from build123d import *

# Parameters (mm, degrees)
SKETCH_1_W          = 200
SKETCH_1_H          = 125
EXTRUDE_1_DEPTH     = 3
SKETCH_2_R          = 4
SKETCH_2_R_2        = 2
EXTRUDE_2_DEPTH     = 28
SKETCH_3_R          = 1.25
CUT_EXTRUDE_1_DEPTH = 10
SKETCH_4_R          = 2
CUT_EXTRUDE_2_DEPTH = 122.203341538
SKETCH_5_R          = 3
EXTRUDE_3_DEPTH     = 8
SKETCH_6_R          = 1.5
CUT_EXTRUDE_3_DEPTH = 8
FILLET_1_R          = 10
RIB_1_REACH         = 205.812
SKETCH_9_WALL_W     = 423.76696313
SKETCH_9_WALL_H     = 5
RIB_2_REACH         = 205.812
SKETCH_10_WALL_W    = 423.76696313
SKETCH_10_WALL_H    = 5
SKETCH_13_R         = 4
EXTRUDE_4_DEPTH     = 8
FILLET_3_R          = 10
SKETCH_14_R         = 1.25
CUT_EXTRUDE_4_DEPTH = 8


with BuildPart() as part:
    # 草图1 → 凸台-拉伸1 (new body)
    with BuildSketch(Plane.XY):
        Rectangle(SKETCH_1_W, SKETCH_1_H)
    extrude(amount=EXTRUDE_1_DEPTH)

    # 草图2 → 凸台-拉伸2 (add)
    with BuildSketch(Plane.XY.offset(3)):
        with Locations(Location((-91.5, 19, 0), (0, 0, 180))):
            Circle(SKETCH_2_R)
        with Locations(Location((-68.5, 19, 0), (0, 0, 180))):
            Circle(SKETCH_2_R_2)
        with Locations(Location((-80, 0, 0), (0, 0, 180))):
            Circle(SKETCH_2_R)
    extrude(amount=EXTRUDE_2_DEPTH)

    # 草图3 → 切除-拉伸1 (cut)
    with BuildSketch(Plane.XY.offset(31)):
        with Locations((-91.5, 19)):
            Circle(SKETCH_3_R)
        with Locations((-68.5, 19)):
            Circle(SKETCH_3_R)
    extrude(amount=-CUT_EXTRUDE_1_DEPTH, mode=Mode.SUBTRACT)

    # 草图4 → 切除-拉伸2 (cut, through all)
    with BuildSketch(Plane.XY.offset(3)):
        with Locations((15.5, 41)):
            Circle(SKETCH_4_R)
        with Locations((15.5, -41)):
            Circle(SKETCH_4_R)
        with Locations((5.5, 41)):
            Circle(SKETCH_4_R)
        with Locations((-4.5, 41)):
            Circle(SKETCH_4_R)
        with Locations((-14.5, -41)):
            Circle(SKETCH_4_R)
        with Locations((-24.5, -41)):
            Circle(SKETCH_4_R)
        with Locations((-4.5, -41)):
            Circle(SKETCH_4_R)
    extrude(amount=-CUT_EXTRUDE_2_DEPTH, mode=Mode.SUBTRACT)

    # 草图5 → 凸台-拉伸3 (add)
    with BuildSketch(Plane.XY.offset(3)):
        with Locations(Location((28.77, 42.73, 0), (0, 0, 180))):
            Circle(SKETCH_5_R)
        with Locations(Location((28.77, -42.73, 0), (0, 0, 180))):
            Circle(SKETCH_5_R)
        with Locations(Location((91.23, -42.73, 0), (0, 0, 180))):
            Circle(SKETCH_5_R)
        with Locations(Location((91.23, 42.73, 0), (0, 0, 180))):
            Circle(SKETCH_5_R)
    extrude(amount=EXTRUDE_3_DEPTH)

    # 草图6 → 切除-拉伸3 (cut)
    with BuildSketch(Plane.XY.offset(11)):
        with Locations((28.77, 42.73)):
            Circle(SKETCH_6_R)
        with Locations((91.23, 42.73)):
            Circle(SKETCH_6_R)
        with Locations((28.77, -42.73)):
            Circle(SKETCH_6_R)
        with Locations((91.23, -42.73)):
            Circle(SKETCH_6_R)
    extrude(amount=-CUT_EXTRUDE_3_DEPTH, mode=Mode.SUBTRACT)

    # 圆角1
    fillet_1_edges = [part.edges().sort_by_distance(p)[0] for p in [
        (100, -62.5, 1.5),
        (-100, -62.5, 1.5),
        (-100, 62.5, 1.5),
        (100, 62.5, 1.5),
    ]]
    fillet(fillet_1_edges, radius=FILLET_1_R)

    # 草图9 wall → 筋1 (add, up to next)
    with BuildSketch(Plane(origin=(-91.5, 28, 8), x_dir=(0, -0.707106781187, 0.707106781187), z_dir=(0, 0.707106781187, 0.707106781187)), mode=Mode.PRIVATE) as rib_1_sk1:
        Rectangle(SKETCH_9_WALL_W, SKETCH_9_WALL_H)
    rib_1_tool1 = extrude(rib_1_sk1.sketch, amount=-RIB_1_REACH, mode=Mode.PRIVATE) - part.part
    add(rib_1_tool1.solids().sort_by_distance((-91.5, 28, 8))[0])

    # 草图10 wall → 筋2 (add, up to next)
    with BuildSketch(Plane(origin=(-91.5, 10, 8), x_dir=(0, -0.707106781187, -0.707106781187), z_dir=(0, -0.707106781187, 0.707106781187)), mode=Mode.PRIVATE) as rib_2_sk1:
        Rectangle(SKETCH_10_WALL_W, SKETCH_10_WALL_H)
    rib_2_tool1 = extrude(rib_2_sk1.sketch, amount=-RIB_2_REACH, mode=Mode.PRIVATE) - part.part
    add(rib_2_tool1.solids().sort_by_distance((-91.5, 10, 8))[0])

    # 草图13 → 凸台-拉伸4 (add)
    with BuildSketch(Plane.XY.offset(3)):
        with Locations(Location((-68.5, 19, 0), (0, 0, 180))):
            Circle(SKETCH_13_R)
    extrude(amount=EXTRUDE_4_DEPTH)

    # 圆角3
    # the kernel refuses this fillet: 10 mm, written as the material it adds along each edge
    with BuildSketch(Plane(origin=(-68.5, 19, 11), x_dir=(-1, 0, 0), z_dir=(0, -1, 0))) as fillet_3_piece_1:
        with BuildLine():
            CenterArc((12, -6), FILLET_3_R, 143.130102354, 36.869897646)
            Line((2, -6), (1.8, -6))
            Line((1.8, -6), (1.8, 0))
            Line((1.8, 0), (2, 0.2))
            ThreePointArc((2, 0.2), (3, 0.2), (3.84, 0.12))
            Line((3.84, 0.12), (4, 0))
        make_face()
    revolve(axis=Axis((-68.5, 19, 11), (0, 0, -1)))

    # 草图14 → 切除-拉伸4 (cut)
    with BuildSketch(Plane.XY.offset(31)):
        with Locations((-80, 0)):
            Circle(SKETCH_14_R)
    extrude(amount=-CUT_EXTRUDE_4_DEPTH, mode=Mode.SUBTRACT)


solid = part.part
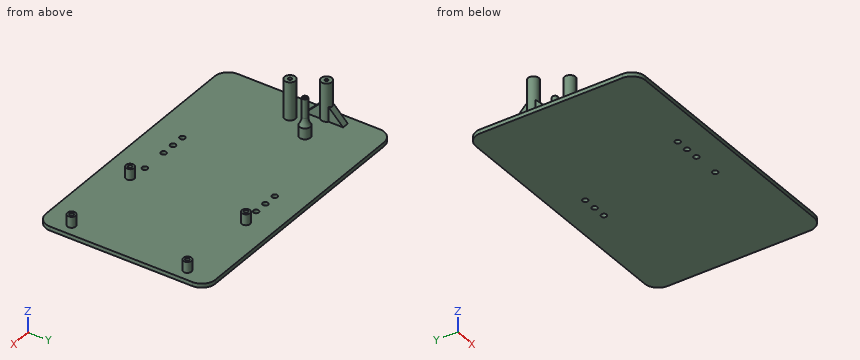
Build history of the part. All positions in model axes, mm. Round coordinates to 2 decimals unless told otherwise and drop trailing zeros. Write each loop counter-clockwise with the first axis right and the second up, starting at its lowest first coordinate (ties: lowest second). Pieces come first, ordered by that corner, then holes. Notation, with made-up numbers: M 64,30 L 112,30 A21 ccw 112,51 Z; hole C -23.5,-33 d8. An arc over 180 degrees is marked long. Answer as a JSON object with one key per item and string values. Group by question number.
(1) Cut at C-C (y = -27). Give the cut face in (x, z).
(2) Cut at A-A (z = 29). Give the cut face in (x, y).
(3) Cut at D-D (x = -35). Give the cut face in (y, z), and give its area (3 significant figures).
(4) Flat gauge pins, fed straight in: pin 1 (1.5 mm diameter, centred on x = 75, y = 16.5, fed in from -Z); pin 2 (12 mm diameter, centred on x = 44, y = -10, fed in from +Z); pin 3 (1.5 mm diameter, centred on x = -91.5, y = 19, fed in from +Z); pin 4 (3.5 mm diameter, centred on y = 30, z = 9.5, fed in from +X). Where does each tip first touch, or does it go through?
(5) Cut at B-B (x = 5.5). Give the cut face in (y, z), and give its area (3 significant figures).
(6) Drill centre lines: L1, parallel to Y at x = 91.23, z = 8.75; L2, parallel to Y at x = -24.5, z = 2.2; L3, parallel to Y at x = -91.5, z = 27.25. Where is each one in solid material? Low to high.
Responses:
{
 "1": {"outline": "M -100,0 L 100,0 L 100,3 L -100,3 Z"},
 "2": {"outline": "C -91.5,19 d8; C -80,0 d8; C -68.5,19 d4; hole C -91.5,19 d2.5; hole C -80,0 d2.5; hole C -68.5,19 d2.5"},
 "3": {"outline": "M -62.5,0 L 62.5,0 L 62.5,3 L -62.5,3 Z", "area": "375 mm2"},
 "4": {"pin 1": "stops at z = 0", "pin 2": "stops at z = 3", "pin 3": "stops at z = 21", "pin 4": "passes through"},
 "5": {"outline": "M -62.5,0 L 39,0 L 39,3 L -62.5,3 Z; M 43,0 L 62.5,0 L 62.5,3 L 43,3 Z", "area": "363 mm2"},
 "6": {"L1": "y = -45.73 to -44.23, -41.23 to -39.73, 39.73 to 41.23, 44.23 to 45.73", "L2": "y = -62.5 to -43, -39 to 62.5", "L3": "y = 15 to 17.75, 20.25 to 23"}
}
